Design review of the part shown in the three views and the two pictorial views. Dimensions are in mm from the part's minimum x, y and z. A direction names the side the tool comes from. Coordinates: 2 decimals unless noted, no trailing zeros. Loops run counter-clockwise (first coordinate to the right, second up) from the corner with the lowest first, then second, coordinate; pieces in that order, holes last. Notation, with made-up numbers: M 40,75 L 86,75 A30 cw 86,99 Z; hole C 47.25,47.5 d1. An arc over 180 degrees is marked long. Use one line per item in the form item = value.
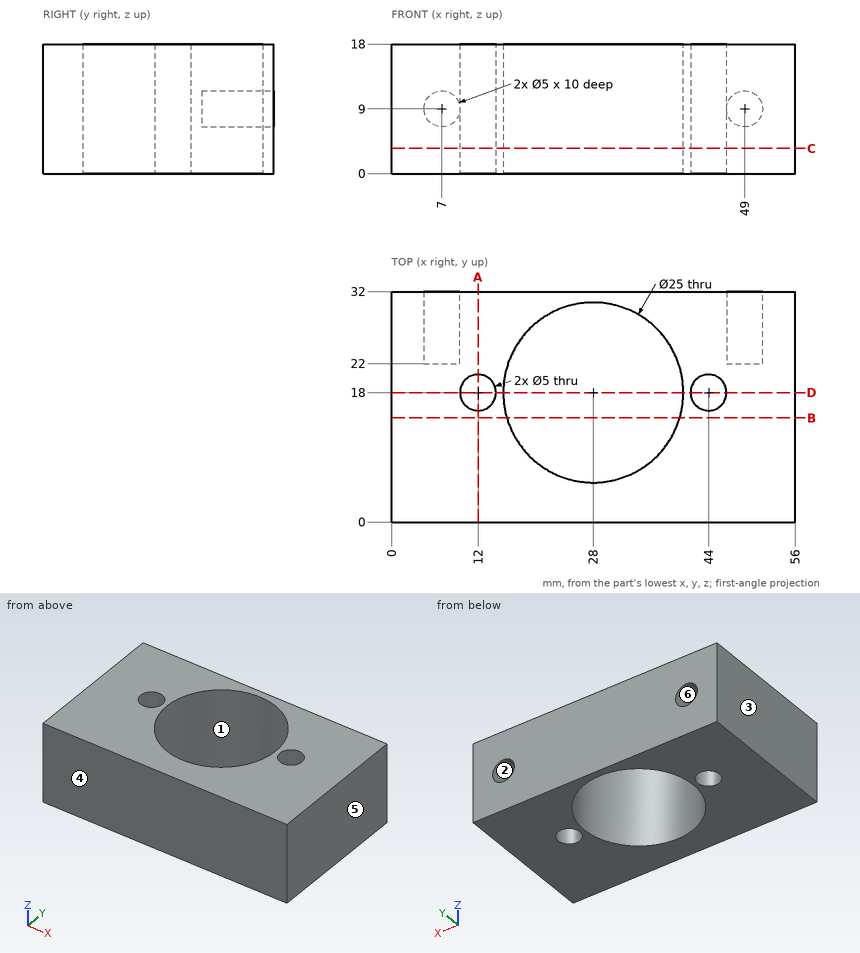
1. Wall thickness on line 1 along Y through (x, z) = (44, 13.75); line 2 along Y through (x, z) = (28, 12); line 3 along Z through (x, y) = (49, 26): over which ranges is each line inside the solid? List them lowest first. Write a range as from..to.
Response values:
line_1 = 0..15.5, 20.5..32
line_2 = 0..5.5, 30.5..32
line_3 = 0..6.5, 11.5..18
2. The part is to be moulded in two halves that separate along X. For the marked faces 1, 2, 3 and 4, say which applies: pulls with the +X half, pulls with the -X half, needs draft (parallel to the pull), parting line crosses it, or undercut.
Response values:
face_1 = undercut
face_2 = undercut
face_3 = pulls with the -X half
face_4 = needs draft
3. Machinability: for the marked faces 5 and 6, which of the approach directions +Z, -Z, +X, -X, +Y, -Y give a long, thin tool a straight path to every point of the face, cutting with its end or side? Answer none if there is none.
Response values:
face_5 = +Z, -Z, +X, +Y, -Y
face_6 = +Y
4. Add section A-A (x = 12). State the section outline as (y, z) points, then the cut area to 3 significant figures.
Response values:
outline = M 0,0 L 15.5,0 L 15.5,18 L 0,18 Z; M 20.5,0 L 32,0 L 32,18 L 20.5,18 Z
area = 486 mm^2
5. Add section D-D (y = 18). State the section outline as (x, z) points, then the cut area to 3 significant figures.
Response values:
outline = M 0,0 L 9.5,0 L 9.5,18 L 0,18 Z; M 14.5,0 L 15.5,0 L 15.5,18 L 14.5,18 Z; M 40.5,0 L 41.5,0 L 41.5,18 L 40.5,18 Z; M 46.5,0 L 56,0 L 56,18 L 46.5,18 Z
area = 378 mm^2
6. Add section B-B (y = 14.5). State the section outline as (x, z) points.
Response values:
outline = M 0,0 L 16,0 L 16,18 L 0,18 Z; M 40,0 L 56,0 L 56,18 L 40,18 Z
7. Insertion check: P1, Ø4, axis at x = 50, z = 10, coming from the +Y side; P2, Ø4.5, axis at x = 44, y = 18, coming from the -Z side. Each pin has a flat end and moves straight along its axis. Give the tip position at first contact, or say it passes through.
Response values:
P1 = 32
P2 = through
8. Add section C-C (z = 3.5). State the section outline as (x, y) points, then the cut area to 3 significant figures.
Response values:
outline = M 0,0 L 56,0 L 56,32 L 0,32 Z; hole C 12,18 d5; hole C 28,18 d25; hole C 44,18 d5
area = 1,260 mm^2
